Design review of the part built by this model. Coordinates are the model's own, in mm. A direction names the side the tool comes from. Round coordinates to 2 decimals unless told otherwise and drop trailing zeros. Order: outer loops, then holes, each group sorted by start corner. A loop starts at its lowest first (then second) coordinate and runs counter-clockwise, first axis right, second up. Notation, with made-up numbers: (50, 70.25) - (101, 70.25) arc R21 ccw to (101, 87.25) - close; hole circle Ø6 at (75.5, 69). An arc over 180 degrees is marked (long way). Write item = value, one per line.
from build123d import *

# Parameters (mm, degrees)
F0_R     = 12
F0_R_2   = 3.75
F1_DEPTH = 2
F3_DEPTH = 5
F5_DEPTH = 12
F6_SIZE2 = 11.99999
F6_SIZE  = 0.49999


# Not quite as in the source:
# - a fillet or chamfer is up to 0.001 mm smaller than in the source, because OpenCascade refuses the exact size


with BuildPart() as f1:
    # F0 (on Top) → F1 (new body)
    with BuildSketch(Plane.XY):
        Circle(F0_R)
        Circle(F0_R_2, mode=Mode.SUBTRACT)
    extrude(amount=F1_DEPTH)

    # F2 (on face) → F3 (join)
    with BuildSketch(Plane.XY.offset(2)):
        with BuildLine():
            Line((-9, -3.5), (-4.5620718977, -3.5))
            ThreePointArc((-4.5620718977, -3.5), (-5.75, 0), (-4.5620718977, 3.5))
            Line((-4.5620718977, 3.5), (-9, 3.5))
            ThreePointArc((-9, 3.5), (-9.7071067812, 3.2071067812), (-10, 2.5))
            Line((-10, 2.5), (-10, 0))
            Line((-10, 0), (-10, -2.5))
            ThreePointArc((-10, -2.5), (-9.7071067812, -3.2071067812), (-9, -3.5))
        make_face()
        with BuildLine():
            Line((-4.5620718977, -3.5), (-1.6039014932, -3.5))
            ThreePointArc((-1.6039014932, -3.5), (-3.0368237131, -2.3664745373), (-3.7858288392, -0.7))
            Line((-3.7858288392, -0.7), (-4, -0.7))
            Line((-4, -0.7), (-4.5464271687, -0.7))
            ThreePointArc((-4.5464271687, -0.7), (-4.6, 0), (-4.5464271687, 0.7))
            Line((-4.5464271687, 0.7), (-3.7858288392, 0.7))
            ThreePointArc((-3.7858288392, 0.7), (-3.0368237131, 2.3664745373), (-1.6039014932, 3.5))
            Line((-1.6039014932, 3.5), (-4.5620718977, 3.5))
            ThreePointArc((-4.5620718977, 3.5), (-5.75, 0), (-4.5620718977, -3.5))
        make_face()
        with BuildLine():
            Line((4.5620718977, -3.5), (1.6039014932, -3.5))
            ThreePointArc((1.6039014932, -3.5), (0, -3.85), (-1.6039014932, -3.5))
            Line((-1.6039014932, -3.5), (-4.5620718977, -3.5))
            ThreePointArc((-4.5620718977, -3.5), (0, -5.75), (4.5620718977, -3.5))
        make_face()
        with BuildLine():
            ThreePointArc((5.75, 0), (5.4449248577, -1.8480512152), (4.5620718977, -3.5))
            Line((4.5620718977, -3.5), (9, -3.5))
            ThreePointArc((9, -3.5), (9.7071067812, -3.2071067812), (10, -2.5))
            Line((10, -2.5), (10, 0))
            Line((10, 0), (10, 2.5))
            ThreePointArc((10, 2.5), (9.7071067812, 3.2071067812), (9, 3.5))
            Line((9, 3.5), (4.5620718977, 3.5))
            ThreePointArc((4.5620718977, 3.5), (5.4449248577, 1.8480512152), (5.75, 0))
        make_face()
        with BuildLine():
            ThreePointArc((3.7858288392, -0.7), (3.0368237131, -2.3664745373), (1.6039014932, -3.5))
            Line((1.6039014932, -3.5), (4.5620718977, -3.5))
            ThreePointArc((4.5620718977, -3.5), (5.4449248577, -1.8480512152), (5.75, 0))
            ThreePointArc((5.75, 0), (5.4449248577, 1.8480512152), (4.5620718977, 3.5))
            Line((4.5620718977, 3.5), (1.6039014932, 3.5))
            ThreePointArc((1.6039014932, 3.5), (3.0368237131, 2.3664745373), (3.7858288392, 0.7))
            Line((3.7858288392, 0.7), (4.5464271687, 0.7))
            ThreePointArc((4.5464271687, 0.7), (4.6, 0), (4.5464271687, -0.7))
            Line((4.5464271687, -0.7), (4, -0.7))
            Line((4, -0.7), (3.7858288392, -0.7))
        make_face()
        with BuildLine():
            Line((-4.5620718977, 3.5), (-1.6039014932, 3.5))
            ThreePointArc((-1.6039014932, 3.5), (0, 3.85), (1.6039014932, 3.5))
            Line((1.6039014932, 3.5), (4.5620718977, 3.5))
            ThreePointArc((4.5620718977, 3.5), (0, 5.75), (-4.5620718977, 3.5))
        make_face()
    extrude(amount=F3_DEPTH)

    # F4 (on face) → F5 (join)
    with BuildSketch(Plane.XY.offset(7)):
        with BuildLine():
            ThreePointArc((4.5620718977, -3.5), (5.4449248577, -1.8480512152), (5.75, 0))
            ThreePointArc((5.75, 0), (5.4449248577, 1.8480512152), (4.5620718977, 3.5))
            ThreePointArc((4.5620718977, 3.5), (0, 5.75), (-4.5620718977, 3.5))
            ThreePointArc((-4.5620718977, 3.5), (-5.75, 0), (-4.5620718977, -3.5))
            ThreePointArc((-4.5620718977, -3.5), (0, -5.75), (4.5620718977, -3.5))
        make_face()
        with BuildLine():
            ThreePointArc((-3.7858288392, 0.7), (0, 3.85), (3.7858288392, 0.7))
            Line((3.7858288392, 0.7), (4.5464271687, 0.7))
            ThreePointArc((4.5464271687, 0.7), (4.6, 0), (4.5464271687, -0.7))
            Line((4.5464271687, -0.7), (3.7858288392, -0.7))
            ThreePointArc((3.7858288392, -0.7), (0, -3.85), (-3.7858288392, -0.7))
            Line((-3.7858288392, -0.7), (-4.5464271687, -0.7))
            ThreePointArc((-4.5464271687, -0.7), (-4.6, 0), (-4.5464271687, 0.7))
            Line((-4.5464271687, 0.7), (-3.7858288392, 0.7))
        make_face(mode=Mode.SUBTRACT)
    extrude(amount=F5_DEPTH)

    # F6 (size 0.5 and 12 in the source; OpenCascade refuses exactly that, so slightly less here)
    f6_edges = [f1.edges().sort_by_distance(p)[0] for p in [
        (-4.562072, -3.5, 19),
    ]]
    f6_side = f1.faces().sort_by_distance((-4.433037, -3.401005, 19))[0]
    chamfer(f6_edges, length=F6_SIZE, length2=F6_SIZE2, reference=f6_side)


solid = f1.part
Item 1: Take a section at A-A, the plane x = 0. State the section outline as (y, z) points.
Data:
outline = (-12, 0) - (-3.75, 0) - (-3.75, 2) - (-3.85, 2) - (-3.85, 19) - (-5.25, 19) - (-5.75, 7) - (-5.75, 2) - (-12, 2) - close; (3.75, 0) - (12, 0) - (12, 2) - (5.75, 2) - (5.75, 7) - (5.25, 19) - (3.85, 19) - (3.85, 2) - (3.75, 2) - close
Item 2: Take a section at D-D, the plane z = 8. State the section outline as (x, y) points, and give its area (3 significant figures).
Data:
outline = circle Ø11.42 at (0, 0); hole (-4.55, -0.7) - (-3.79, -0.7) arc R3.85 ccw to (3.79, -0.7) - (4.55, -0.7) arc R4.6 ccw to (4.55, 0.7) - (3.79, 0.7) arc R3.85 ccw to (-3.79, 0.7) - (-4.55, 0.7) arc R4.6 ccw to start
area = 53.7 mm2
Item 3: For faces 5 (the face through (-7, 3.5, 4)), 6 (the face through (-2.8, -5.2, 2)), 7 (the face through (9.699, -3.215, 4.465)), 8 (the face through (-10, 0, 4)), list the 3-axis set-ups (+Z, -Z, +X, -X, +Y, -Y) from which the entire face can be reached by the end or side of a thin tool; tool diameter is ignored.
Data:
face_5 = +Z, -X, +Y
face_6 = +Z
face_7 = +Z, +X, -Y
face_8 = +Z, -X, +Y, -Y
Item 4: Take a section at B-B, the plane z = 5.5. State the section outline as (x, y) points.
Data:
outline = (-10, -2.5) arc R1 ccw to (-9, -3.5) - (-4.56, -3.5) arc R5.75 ccw to (4.56, -3.5) - (9, -3.5) arc R1 ccw to (10, -2.5) - (10, 2.5) arc R1 ccw to (9, 3.5) - (4.56, 3.5) arc R5.75 ccw to (-4.56, 3.5) - (-9, 3.5) arc R1 ccw to (-10, 2.5) - close; hole (-4.55, -0.7) - (-3.79, -0.7) arc R3.85 ccw to (3.79, -0.7) - (4.55, -0.7) arc R4.6 ccw to (4.55, 0.7) - (3.79, 0.7) arc R3.85 ccw to (-3.79, 0.7) - (-4.55, 0.7) arc R4.6 ccw to start
Item 5: Take a section at C-C, the plane y = -6.75. State the section outline as (x, z) points, and give its area (3 significant figures).
Data:
outline = (-9.92, 0) - (9.92, 0) - (9.92, 2) - (-9.92, 2) - close
area = 39.7 mm2
Item 6: For line 1 along Y through (x, z) = (0, 1.1); line 2 along Y through (x, z) = (-8, 2.25); line 3 along Y through (x, z) = (0.75, 6.5), list the stretches that pass through material, from the lowest coordinate up. Write a range as [from, to].
Data:
line_1 = [-12, -3.75], [3.75, 12]
line_2 = [-3.5, 3.5]
line_3 = [-5.7, -3.78], [3.78, 5.7]
Item 7: Insertion check: P1, Ø0.8, axis at x = -4.5, z = 12, coming from the -Y side; P2, Ø3.5, axis at x = 6, z = 5, coming from the -Y side; P3, Ø1.6, axis at x = 8, y = -0.5, coming from the +Z side. Each pin has a flat end and moves straight along its axis. Give the tip position at first contact, or say it passes through.
Data:
P1 = -3.73
P2 = -3.87
P3 = 7
Item 8: The part is to be moulded in two halves that separate along Y. For faces 1 (the face through (-4.6, 0, 10.4)), 2 (the face through (-11.99, 0.53, 0.99)), 3 (the face through (-3, 3, 0)), 4 (the face through (4.6, 0, 10.4)), say which applies: +Y half, -Y half, draft (parallel to the pull), parting line (faces both ways), or undercut.
Data:
face_1 = undercut
face_2 = parting line
face_3 = draft
face_4 = undercut
